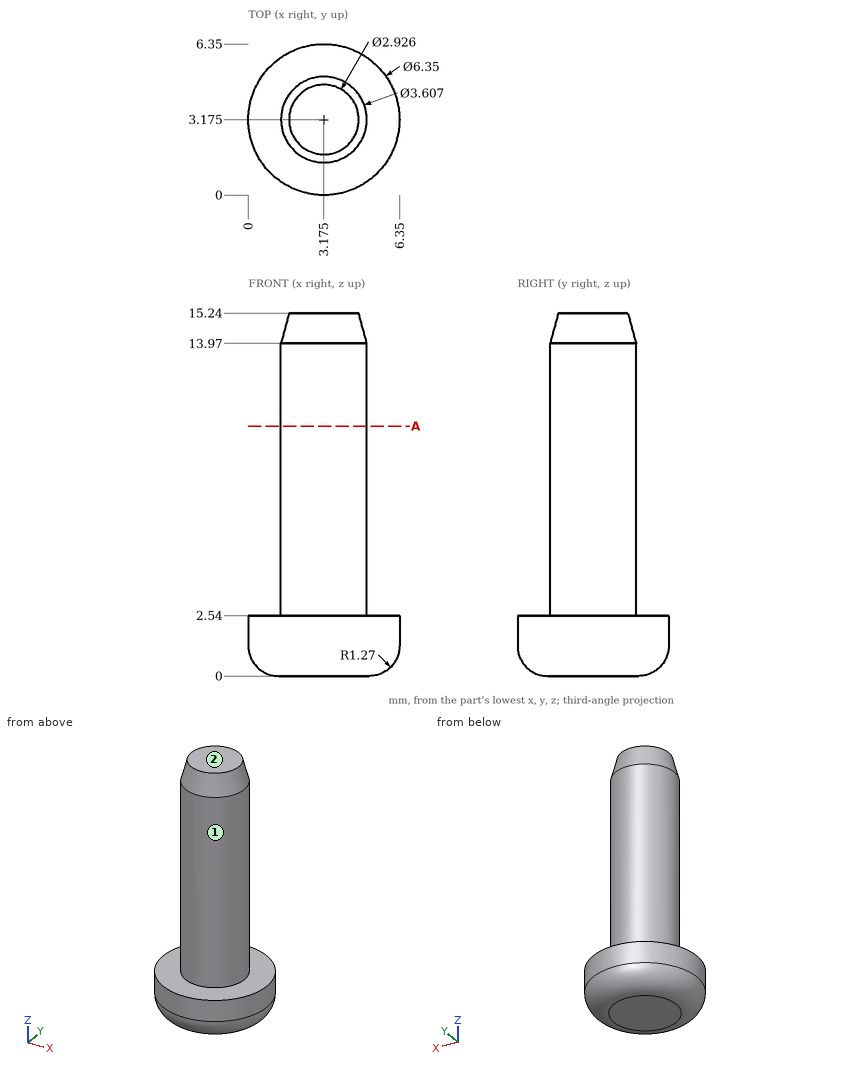
Could you check a few things on this drawing? It's one solid part, dimensions in mm from its lowest x, y, z. A direction names the side the tool comes from. Coordinates: 2 decimals unless noted, no trailing zeros. Write each loop counter-clockwise with the first axis right and the second up, starting at its lowest first coordinate (ties: lowest second). Pieces come first, ordered by that corner, then holes.
1) If we section it at A-A (z = 10.5): List the corners of the cut face in (x, y) for me (1 decimal), plus the area to 3 significant figures.
Filled in:
outline: circle Ø3.6 at (3.2, 3.2)
area: 10.2 mm2
2) I'm going to push flat-ended pins straight in: pin 1 (3 mm diameter, centred on y = 3, z = 11, fed in from +X); pin 2 (1.5 mm diameter, centred on x = 2.5, z = 4.5, fed in from -Y); pin 3 (1.5 mm diameter, centred on x = 5.5, z = 13, fed in from +Y). Where does each tip first touch, or does it pass through?
Filled in:
pin 1: stops at x = 4.98
pin 2: stops at y = 1.37
pin 3: stops at y = 4.05
3) Which directions (+Z, -Z, +X, -X, +Y, -Y) give clear straight access to the entire face, cutting with the end or side of a thin tool? Please do the marked faces 1 and 2.
Filled in:
face 1: +Z
face 2: +Z, +X, -X, +Y, -Y
4) If I drill on line 1 (Z direction, x = 2.75, y = 5); line 2 (Y direction, x = 1.75, z = 5.75); line 3 (Y direction, x = 2.25, z = 8), over which ranges is the centre line in solid material (lowest first)?
Filled in:
line 1: z = 0 to 2.54
line 2: y = 2.07 to 4.28
line 3: y = 1.63 to 4.72
